Could you check a few things on this model? Use its own coordinates, in mm. Give positions to 0.01 mm unless a question says otherwise; leave off trailing zeros. Order: outer loops, then holes, each group sorted by start corner. A loop starts at its lowest first (then second) coordinate and runs counter-clockwise, first axis right, second up.
(1) If I drill on probe 1 along Y at (x, z) = (0, 1.2); probe 2 along Y at (x, z) = (1, 1.25); probe 3 along X at (y, z) = (9, 0.15), over which ranges is the centre line in solid material (lowest first)?
(2) Imagine slicing it at B-B, the plane z = 1.1. Write out the boundary of the cut face in (x, y), then the cut area to 3 significant figures.
(3) Imagine slicing it at C-C, the plane y = -10. Write out the boundary of the cut face in (x, z).
(4) Will this pin go through, and if not, where does the flat tip stop? pin 1 (4.5 mm diameter, centred on x = 0, y = 30, fed in from +Z).
(5) If we mould it in two halves opening along X, with no side actions, what happens to faces 1 (the flat face through (0, 1, 2)), 2 (the cylindrical face through (0.358, 12.727, 0.986)), 3 (the flat face through (-10, -1, 1)), 4 (the cylindrical face through (2.027, -8.141, 0.986))? For each: released by +X, released by -X, zero draft, split by the parting line, or undercut.
(6) Imagine slicing it at D-D, the plane y = -28.5. Write out the boundary of the cut face in (x, z).
(7) Imagine slicing it at A-A, the plane x = 0. Write out the boundary of the cut face in (y, z), then the cut area to 3 significant figures.
from build123d import *

# Parameters (mm, degrees)
SKETCH_1_W        = 20
SKETCH_1_H        = 80
EXTRUDE_1_DEPTH   = 2
CHAMFER_1_SIZE    = 2
HOLE_WIZARD_M51_D = 5.5


with BuildPart() as part:
    # Эскиз1 → Бобышка-Вытянуть1 (new body)
    with BuildSketch(Plane.XY):
        Rectangle(SKETCH_1_W, SKETCH_1_H)
    extrude(amount=EXTRUDE_1_DEPTH)

    # Фаска1
    chamfer_1_edges = [part.edges().sort_by_distance(p)[0] for p in [
        (10, -40, 1),
        (-10, -40, 1),
        (-10, 40, 1),
        (10, 40, 1),
    ]]
    chamfer(chamfer_1_edges, length=CHAMFER_1_SIZE)

    # Отверстие с зазором M51 (through all)
    with Locations(Plane.XY.offset(2)):
        with Locations((0, -30), (0, 30), (0, 10), (0, -10)):
            Hole(HOLE_WIZARD_M51_D / 2)


solid = part.part
Answer block:
1. probe 1: y = -40 to -32.75, -27.25 to -12.75, -7.25 to 7.25, 12.75 to 27.25, 32.75 to 40
1. probe 2: y = -40 to -32.56, -27.44 to -12.56, -7.44 to 7.44, 12.56 to 27.44, 32.56 to 40
1. probe 3: x = -10 to -2.56, 2.56 to 10
2. outline: (-10, -38) - (-8, -40) - (8, -40) - (10, -38) - (10, 38) - (8, 40) - (-8, 40) - (-10, 38) - close; hole circle Ø5.5 at (0, -30); hole circle Ø5.5 at (0, -10); hole circle Ø5.5 at (0, 10); hole circle Ø5.5 at (0, 30)
2. area: 1,500 mm2
3. outline: (-10, 0) - (-2.75, 0) - (-2.75, 2) - (-10, 2) - close; (2.75, 0) - (10, 0) - (10, 2) - (2.75, 2) - close
4. pin 1: passes through
5. face 1: zero draft
5. face 2: undercut
5. face 3: released by -X
5. face 4: undercut
6. outline: (-10, 0) - (-2.3, 0) - (-2.3, 2) - (-10, 2) - close; (2.3, 0) - (10, 0) - (10, 2) - (2.3, 2) - close
7. outline: (-40, 0) - (-32.75, 0) - (-32.75, 2) - (-40, 2) - close; (-27.25, 0) - (-12.75, 0) - (-12.75, 2) - (-27.25, 2) - close; (-7.25, 0) - (7.25, 0) - (7.25, 2) - (-7.25, 2) - close; (12.75, 0) - (27.25, 0) - (27.25, 2) - (12.75, 2) - close; (32.75, 0) - (40, 0) - (40, 2) - (32.75, 2) - close
7. area: 116 mm2
